Verification items for the finished model (mm, model axes). Face numbers are marked on the shaded views. A direction names the side the tool comes from. Round coordinates to 2 decimals unless told otherwise and drop trailing zeros. Order: outer loops, then holes, each group sorted by start corner. A loop starts at its lowest first (then second) coordinate and runs counter-clockwise, first axis right, second up. Notation, with made-up numbers: (71.25, -19) -> (108.25, -19) arc R12 cw to (108.25, -2) -> close; hole circle Ø4 at (60.25, 77.5). An arc over 180 degrees is marked (long way). Put each result on its own line as item: value.
from build123d import *

# Parameters (mm, degrees)
F0_R     = 12.7
F0_R_2   = 11.049
F1_DEPTH = 4.7625
F3_DEPTH = 4.7625
F4_R     = 4.76249
F5_R     = 4.76249


# Not quite as in the source:
# - a fillet or chamfer is up to 0.001 mm smaller than in the source, because OpenCascade refuses the exact size


with BuildPart() as f1:
    # F0 (on Top) → F1 (new body, symmetric)
    with BuildSketch(Plane.XY):
        Circle(F0_R)
        Circle(F0_R_2, mode=Mode.SUBTRACT)
    extrude(amount=F1_DEPTH, both=True)

    # F2 (on Top) → F3 (join, symmetric)
    with BuildSketch(Plane.XY):
        with BuildLine():
            ThreePointArc((-10.3695065778, -7.3323484187), (-12.7, 0), (-10.3695065778, 7.3323484187))
            Line((-10.3695065778, 7.3323484187), (-19.05, 7.3323484187))
            Line((-19.05, 7.3323484187), (-31.75, 14.6646968374))
            Line((-31.75, 14.6646968374), (-44.45, 7.3323484187))
            Line((-44.45, 7.3323484187), (-44.45, -7.3323484187))
            Line((-44.45, -7.3323484187), (-31.75, -14.6646968374))
            Line((-31.75, -14.6646968374), (-19.05, -7.3323484187))
            Line((-19.05, -7.3323484187), (-10.3695065778, -7.3323484187))
        make_face()
        with BuildLine():
            Line((44.45, -7.3323484187), (44.45, 7.3323484187))
            Line((44.45, 7.3323484187), (31.75, 14.6646968374))
            Line((31.75, 14.6646968374), (19.05, 7.3323484187))
            Line((19.05, 7.3323484187), (10.3695065778, 7.3323484187))
            ThreePointArc((10.3695065778, 7.3323484187), (12.7, 0), (10.3695065778, -7.3323484187))
            Line((10.3695065778, -7.3323484187), (19.05, -7.3323484187))
            Line((19.05, -7.3323484187), (31.75, -14.6646968374))
            Line((31.75, -14.6646968374), (44.45, -7.3323484187))
        make_face()
    extrude(amount=F3_DEPTH, both=True)

    # F4 (radius 4.7625 in the source; OpenCascade refuses exactly that, so slightly less here)
    f4_edges = [f1.edges().sort_by_distance(p)[0] for p in [
        (38.1, -10.998523, 4.7625),
        (44.45, 0, 4.7625),
        (25.4, -10.998523, 4.7625),
        (14.709753, -7.332348, 4.7625),
        (14.709753, 7.332348, 4.7625),
        (25.4, 10.998523, 4.7625),
        (38.1, 10.998523, 4.7625),
        (14.709753, -7.332348, -4.7625),
        (25.4, -10.998523, -4.7625),
        (38.1, -10.998523, -4.7625),
        (44.45, 0, -4.7625),
        (14.709753, 7.332348, -4.7625),
        (25.4, 10.998523, -4.7625),
        (38.1, 10.998523, -4.7625),
    ]]
    fillet(f4_edges, radius=F4_R)

    # F5 (radius 4.7625 in the source; OpenCascade refuses exactly that, so slightly less here)
    f5_edges = [f1.edges().sort_by_distance(p)[0] for p in [
        (-38.1, 10.998523, 4.7625),
        (-25.4, 10.998523, 4.7625),
        (-14.709753, 7.332348, 4.7625),
        (-14.709753, -7.332348, 4.7625),
        (-25.4, -10.998523, 4.7625),
        (-38.1, -10.998523, 4.7625),
        (-44.45, 0, -4.7625),
        (-44.45, 0, 4.7625),
        (-25.4, -10.998523, -4.7625),
        (-38.1, -10.998523, -4.7625),
        (-14.709753, -7.332348, -4.7625),
        (-14.709753, 7.332348, -4.7625),
        (-25.4, 10.998523, -4.7625),
        (-38.1, 10.998523, -4.7625),
    ]]
    fillet(f5_edges, radius=F5_R)


solid = f1.part
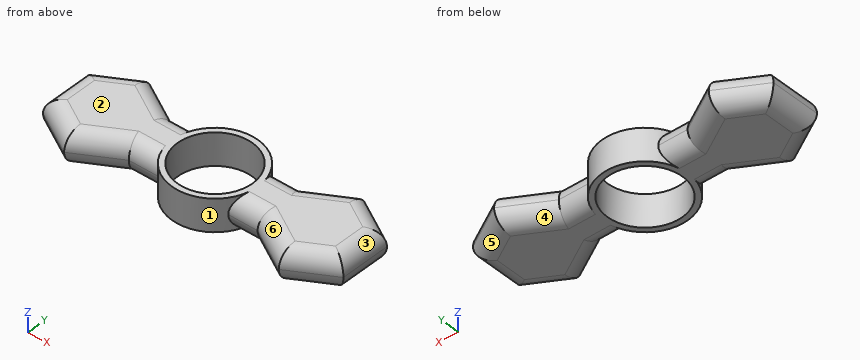
Item 1: Section check B-B on x = 0. Record the boundary of the cut face in (y, z), then the cut area to 3 significant figures.
Check sheet entries:
outline: (-12.7, -4.76) -> (-11.05, -4.76) -> (-11.05, 4.76) -> (-12.7, 4.76) -> close; (11.05, -4.76) -> (12.7, -4.76) -> (12.7, 4.76) -> (11.05, 4.76) -> close
area: 31.5 mm^2
Item 2: Tool access check on the marked faces 4, 5 and 6. Record the directions out of +Z, -Z, +X, -X, +Y, -Y that give a thin tool (end or side, any length) a straight path to the whole face; none if there is none.
Check sheet entries:
face 4: -Z, +Y
face 5: -Z, +X, +Y
face 6: +Z, -Y
Item 3: Section check C-C on z = 1.75. Record the boundary of the cut face in (x, y), then the cut area to 3 significant figures.
Check sheet entries:
outline: (-44.12, -7.14) -> (-31.75, -14.28) -> (-19.14, -7) -> (-10.6, -7) arc R12.7 ccw to (10.6, -7) -> (19.14, -7) -> (31.75, -14.28) -> (44.12, -7.14) -> (44.12, 7.14) -> (31.75, 14.28) -> (19.14, 7) -> (10.6, 7) arc R12.7 ccw to (-10.6, 7) -> (-19.14, 7) -> (-31.75, 14.28) -> (-44.12, 7.14) -> close; hole circle Ø22.1 at (0, 0)
area: 1,390 mm^2
Item 4: Release check for a two-part mould opening along X. For the marked faces 1, 2 and 3 record: +X half, -X half, draft (parallel to the pull), parting line (faces both ways), or undercut.
Check sheet entries:
face 1: undercut
face 2: draft
face 3: +X half
Item 5: Gauge pin test, flat ends, axial feed: pin 1 Ø1.5 at (x, z) = (17, 2.5) entering from -Y; pin 2 Ø5 at (x, z) = (24.5, 2) entering from -Y; pin 3 Ø3 at (y, z) = (-3.5, 3.5) entering from -X. Record the tip position at first contact, or that the pin passes through.
Check sheet entries:
pin 1: stops at y = -7
pin 2: stops at y = -11.68
pin 3: stops at x = -44.01
Item 6: Material ranges on L1, parallel to X at y = -7.5, z = 1.5; L2, parallel to X at y = -0.5, z = -3.5; L3, parallel to X at y = -4, z = -1, recorded low to high. Write a range as [from, to].
Check sheet entries:
L1: x = [-43.67, -19.83], [-10.25, -8.11], [8.11, 10.25], [19.83, 43.67]
L2: x = [-42.92, -11.04], [11.04, 42.92]
L3: x = [-44.34, -10.3], [10.3, 44.34]
